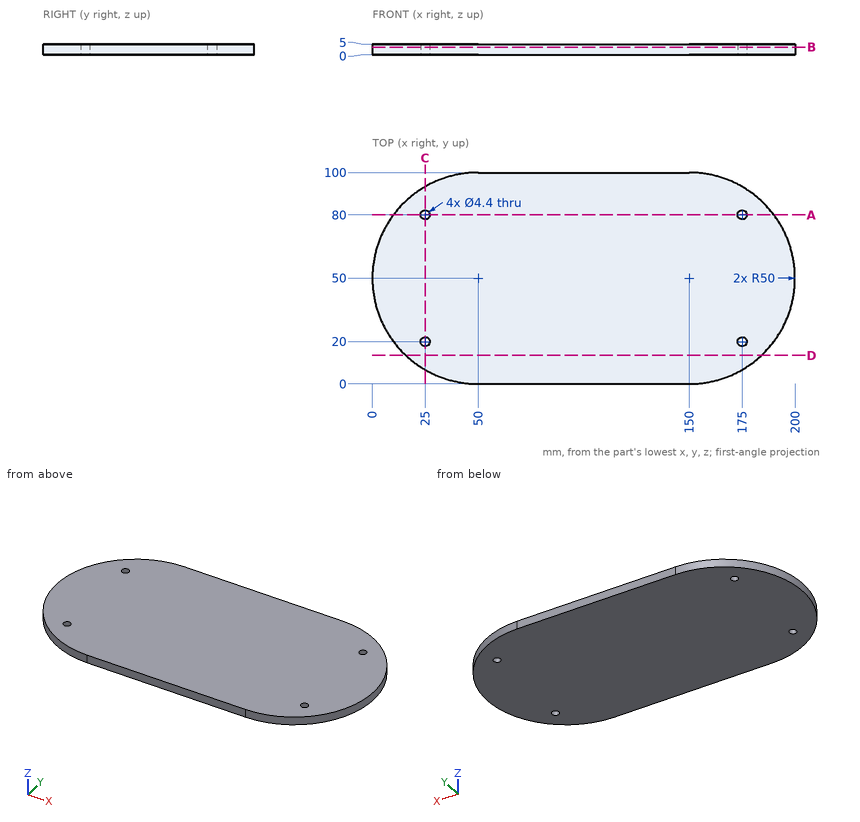
Drawing for the job (mm, zero at the part's lowest x, y, z). Round coordinates to 2 decimals unless told otherwise and drop trailing zeros. Write each loop counter-clockwise with the first axis right and the second up, starting at its lowest first coordinate (ties: lowest second). Pieces come first, ordered by that corner, then holes.
Item 1: Band-saw the part on B-B on z = 3.55. Write the cut outline in (x, y).
Filled in:
outline: (50, 0) - (150, 0) arc R50 ccw to (150, 100) - (50, 100) arc R50 ccw to start; hole circle Ø4.4 at (25, 20); hole circle Ø4.4 at (25, 80); hole circle Ø4.4 at (175, 20); hole circle Ø4.4 at (175, 80)
Item 2: Band-saw the part on D-D on y = 13.5. Write the cut outline in (x, z), then the cut area to 3 significant figures.
Filled in:
outline: (15.83, 0) - (184.17, 0) - (184.17, 5) - (15.83, 5) - close
area: 842 mm2
Item 3: Drop a flat-ended pin along its axis: pin 1 Ø2 at (y, z) = (79, 4) entering from -X. Give the stop position or say it passes through.
Filled in:
pin 1: stops at x = 8.58
Item 4: Band-saw the part on C-C on x = 25. Write the cut outline in (y, z), then the cut area to 3 significant figures.
Filled in:
outline: (6.7, 0) - (17.8, 0) - (17.8, 5) - (6.7, 5) - close; (22.2, 0) - (77.8, 0) - (77.8, 5) - (22.2, 5) - close; (82.2, 0) - (93.3, 0) - (93.3, 5) - (82.2, 5) - close
area: 389 mm2
Item 5: Drill centre lines: L1, parallel to Y at x = 25.5, z = 4.65; L2, parallel to Y at x = 25, z = 1.45; L3, parallel to Y at x = 179, z = 4.1. Where is each one in solid material? Low to high.
Filled in:
L1: y = 6.41 to 17.86, 22.14 to 77.86, 82.14 to 93.59
L2: y = 6.7 to 17.8, 22.2 to 77.8, 82.2 to 93.3
L3: y = 9.27 to 90.73
Item 6: Band-saw the part on A-A on y = 80. Write the cut outline in (x, z), then the cut area to 3 significant figures.
Filled in:
outline: (10, 0) - (22.8, 0) - (22.8, 5) - (10, 5) - close; (27.2, 0) - (172.8, 0) - (172.8, 5) - (27.2, 5) - close; (177.2, 0) - (190, 0) - (190, 5) - (177.2, 5) - close
area: 856 mm2
